Geometry check sheet. Reference: the model listing, model coordinates, mm. A direction names the side the tool comes from. Round coordinates to 2 decimals unless told otherwise and drop trailing zeros. Loops run counter-clockwise (first coordinate to the right, second up) from the corner with the lowest first, then second, coordinate; pieces in that order, holes last. Notation, with made-up numbers: M 18.25,44 L 35.25,44 A21 cw 35.25,58 Z; hole C -32,-5.5 d5. An arc over 180 degrees is marked long. Write item = value, one per line.
from build123d import *

# Parameters (mm, degrees)
F0_R     = 92.815735633
F0_R_2   = 86.0311555183
F1_DEPTH = 25.4
F0_R_3   = 38.21812987
F2_R     = 92.71
F3_DEPTH = 3.175


with BuildPart() as f1:
    # F0 (on Front) → F1 (new body)
    with BuildSketch(Plane.XZ):
        Circle(F0_R)
        Circle(F0_R_2, mode=Mode.SUBTRACT)
    extrude(amount=F1_DEPTH)



with BuildPart() as f1b:
    # F0 (on Front) → F1, piece 2 (new body)
    with BuildSketch(Plane.XZ):
        with BuildLine():
            Line((50.8, 59.6587392047), (-50.8, 59.6587392047))
            Line((-50.8, 59.6587392047), (-50.8, 47.720739051))
            Line((-50.8, 47.720739051), (-24.8520022743, 47.720739051))
            ThreePointArc((-24.8520022743, 47.720739051), (-50.7246708671, 0.8577388972), (-24.8520022743, -46.0052612565))
            Line((-24.8520022743, -46.0052612565), (-50.8, -46.0052612565))
            Line((-50.8, -46.0052612565), (-50.8, -57.6892601803))
            Line((-50.8, -57.6892601803), (50.8, -57.6892601803))
            Line((50.8, -57.6892601803), (50.8, -46.0052612565))
            Line((50.8, -46.0052612565), (25.9479958039, -46.0052612565))
            ThreePointArc((25.9479958039, -46.0052612565), (50.9828195519, 0.8577388972), (25.9479958039, 47.720739051))
            Line((25.9479958039, 47.720739051), (50.8, 47.720739051))
            Line((50.8, 47.720739051), (50.8, 59.6587392047))
        make_face()
        Circle(F0_R_3, mode=Mode.SUBTRACT)
    extrude(amount=F1_DEPTH)


with BuildPart() as f1_1:
    add(f1.part)

    add(f1b.part)  # F3 merges F1b
    # F2 (on face) → F3 (join)
    with BuildSketch(Plane(origin=(0, 0, 0), x_dir=(-1, 0, 0), z_dir=(0, 1, 0))):
        Circle(F2_R)
    extrude(amount=F3_DEPTH)


solid = f1_1.part
(1) Material ranges on line 1 along Z through (x, y) = (0, -15.75); line 2 along Z through (x, y) = (-12.5, -8.75); line 3 along X through (y, z) = (-20, 42.5), recorded low to high. Write a range as from..to.
Result set:
line_1 = -92.82..-86.03, -57.69..-38.22, 38.22..59.66, 86.03..92.82
line_2 = -91.97..-85.12, -57.69..-36.12, 36.12..59.66, 85.12..91.97
line_3 = -82.51..-74.8, -31.85..32.61, 74.8..82.51
(2) Sectioned sample at D-D on x = -79. Record the cut outline in (y, z) (3 decimals), then the cut area to 3 significant figures.
Result set:
outline = M -25.4,-48.721 L 0,-48.721 L 0,-48.52 L 3.175,-48.52 L 3.175,48.52 L 0,48.52 L 0,48.721 L -25.4,48.721 L -25.4,34.064 L 0,34.064 L 0,-34.064 L -25.4,-34.064 Z
area = 1,050 mm2
(3) Sectioned sample at C-C on z = 16. Record the cut outline in (x, y) (3 decimals), then the cut area to 3 significant figures.
Result set:
outline = M -91.426,-25.4 L -84.53,-25.4 L -84.53,0 L -48.614,0 L -48.614,-25.4 L -34.708,-25.4 L -34.708,0 L 34.708,0 L 34.708,-25.4 L 48.911,-25.4 L 48.911,0 L 84.53,0 L 84.53,-25.4 L 91.426,-25.4 L 91.426,0 L 91.319,0 L 91.319,3.175 L -91.319,3.175 L -91.319,0 L -91.426,0 Z
area = 1,640 mm2
(4) Depth check by flat-ended pin: pin 1 Ø2 at (x, z) = (-63, -51) entering from -Y; pin 2 Ø4 at (x, y) = (24.5, -21) entering from +Z; pin 3 Ø1.5 at (y, z) = (-10.5, -41) entering from -X. Enter the tip coordinate at first touch or a pass-through.
Result set:
pin_1 = 0
pin_2 = 90.05
pin_3 = -83.63
(5) Sectioned sample at B-B on x = 0. Record the cut outline in (y, z) (3 decimals).
Result set:
outline = M -25.4,-92.816 L 0,-92.816 L 0,-92.71 L 3.175,-92.71 L 3.175,92.71 L 0,92.71 L 0,92.816 L -25.4,92.816 L -25.4,86.031 L 0,86.031 L 0,59.659 L -25.4,59.659 L -25.4,38.218 L 0,38.218 L 0,-38.218 L -25.4,-38.218 L -25.4,-57.689 L 0,-57.689 L 0,-86.031 L -25.4,-86.031 Z
(6) Release check for a two-part mould opening along Z. For faces 1 (the flat face through (27, -25.4, -82)), 2 (the flat face through (-50.8, -13, 54)), 3 (the cylindrical face through (-85.64, 1.57, -35.51)) record: released by +Z, released by -Z, zero draft, split by the parting line, or undercut.
Result set:
face_1 = zero draft
face_2 = undercut
face_3 = split by the parting line
(7) Tool access check on faces 4 (the cylindrical face through (36.453, -12.522, 11.48)), 5 (the flat face through (11, -25.4, -37)). Record the directions out of +Z, -Z, +X, -X, +Y, -Y that give a thin tool (end or side, any length) a straight path to the whole face; none if there is none.
Result set:
face_4 = -Y
face_5 = +Z, -Z, +X, -X, -Y
(8) Sectioned sample at A-A on y = -22.5. Record the cut outline in (x, z).
Result set:
outline = C 0,0 d185.63; M -50.8,-57.69 L 50.8,-57.69 L 50.8,-46.01 L 25.95,-46.01 A56.38 ccw 25.95,47.72 L 50.8,47.72 L 50.8,59.66 L -50.8,59.66 L -50.8,47.72 L -24.85,47.72 A55.38 ccw -24.85,-46.01 L -50.8,-46.01 Z; hole C 0,0 d172.06; hole C 0,0 d76.44
